```python
from build123d import *

# Parameters (mm, degrees)
SKETCH1_W            = 1447.8
SKETCH1_H            = 215.9
BOSS_EXTRUDE1_DEPTH  = 6.35
SKETCH2_R            = 82.55
CUT_EXTRUDE1_DEPTH   = 7.35
LPATTERN1_COUNT      = 7
LPATTERN1_PITCH      = 203.2
FILLET1_R            = 25.4
CUT_EXTRUDE2_DEPTH   = 7.35
LPATTERN2_COUNT      = 2
LPATTERN2_PITCH      = 406.4
MIRROR1_COPY_1_DEPTH = 7.35
SKETCH4_R            = 3.175
CUT_EXTRUDE3_DEPTH   = 7.35


with BuildPart() as part:
    # Sketch1 → Boss-Extrude1 (new body)
    with BuildSketch(Plane.XY):
        Rectangle(SKETCH1_W, SKETCH1_H)
    extrude(amount=BOSS_EXTRUDE1_DEPTH)

    # Sketch2 → Cut-Extrude1 (cut, through all)
    with BuildSketch(Plane.XY.offset(6.35)):
        with Locations((-609.6, 0)):
            Circle(SKETCH2_R)
    cut_extrude1 = extrude(amount=-CUT_EXTRUDE1_DEPTH, mode=Mode.SUBTRACT)

    # LPattern1: Cut-Extrude1 ×7
    with Locations(*[(i * LPATTERN1_PITCH, 0, 0) for i in range(1, LPATTERN1_COUNT)]):
        add(cut_extrude1, mode=Mode.SUBTRACT)

    # Fillet1
    fillet1_edges = [part.edges().sort_by_distance(p)[0] for p in [
        (-723.9, 107.95, 3.175),
        (723.9, 107.95, 3.175),
    ]]
    fillet(fillet1_edges, radius=FILLET1_R)

    # Sketch3 → Cut-Extrude2 (cut, through all)
    with BuildSketch(Plane.XY.offset(6.35)):
        with BuildLine():
            Line((-706.4375, 50.8), (-706.4375, 31.75))
            ThreePointArc((-706.4375, 31.75), (-711.2, 26.9875), (-715.9625, 31.75))
            Line((-715.9625, 31.75), (-715.9625, 50.8))
            ThreePointArc((-715.9625, 50.8), (-711.2, 55.5625), (-706.4375, 50.8))
        make_face()
    cut_extrude2 = extrude(amount=-CUT_EXTRUDE2_DEPTH, mode=Mode.SUBTRACT)

    # LPattern2: Cut-Extrude2 ×2
    with Locations(*[(i * LPATTERN2_PITCH, 0, 0) for i in range(1, LPATTERN2_COUNT)]):
        add(cut_extrude2, mode=Mode.SUBTRACT)

    # Mirror1: Cut-Extrude2 across plane
    add(cut_extrude2.mirror(Plane(origin=(0, 0, 0), x_dir=(0, 0, 1), z_dir=(1, 0, 0))), mode=Mode.SUBTRACT)

    # Mirror1 copy 1 sketch → Mirror1 copy 1 (cut, through all)
    with BuildSketch(Plane(origin=(-406.4, 0, 6.35), x_dir=(-1, 0, 0), z_dir=(0, 0, 1))):
        with BuildLine():
            Line((-706.4375, -50.8), (-706.4375, -31.75))
            ThreePointArc((-706.4375, -31.75), (-711.2, -26.9875), (-715.9625, -31.75))
            Line((-715.9625, -31.75), (-715.9625, -50.8))
            ThreePointArc((-715.9625, -50.8), (-711.2, -55.5625), (-706.4375, -50.8))
        make_face()
    extrude(amount=-MIRROR1_COPY_1_DEPTH, mode=Mode.SUBTRACT)

    # Sketch4 → Cut-Extrude3 (cut, through all)
    with BuildSketch(Plane.XY.offset(6.35)):
        with Locations((-698.5, 19.05)):
            Circle(SKETCH4_R)
        with Locations((-317.5, 19.05)):
            Circle(SKETCH4_R)
        with Locations((-292.1, 19.05)):
            Circle(SKETCH4_R)
        with Locations((-698.5, -82.55)):
            Circle(SKETCH4_R)
        with Locations((-317.5, -82.55)):
            Circle(SKETCH4_R)
        with Locations((-292.1, -82.55)):
            Circle(SKETCH4_R)
    cut_extrude3 = extrude(amount=-CUT_EXTRUDE3_DEPTH, mode=Mode.SUBTRACT)

    # Mirror2: Cut-Extrude3 across plane
    add(cut_extrude3.mirror(Plane(origin=(0, 0, 0), x_dir=(0, 0, 1), z_dir=(1, 0, 0))), mode=Mode.SUBTRACT)


solid = part.part
```
Read the model definition and answer for the solid it produces. Units are mm, in the model's axes. Coordinates: 2 decimals unless noted, no trailing zeros. Write each loop counter-clockwise with the first axis right and the second up, starting at its lowest first coordinate (ties: lowest second). Pieces come first, ordered by that corner, then holes. Notation, with made-up numbers: (19, 22.5) -> (76, 22.5) arc R11 ccw to (76, 38.5) -> close; hole circle Ø1 at (46.25, -27.5). An arc over 180 degrees is marked (long way). Answer as a JSON object with one key per item and string values.
Q1. The part is cut by section B-B on y = -43. Give the number of separate pieces and of enclosed holes in the cut face, then the cut area to 3 significant figures.
The answers:
{"separate pieces": "8", "enclosed holes": "0", "area": "2,930 mm2"}
Q2. The part is cut by section A-A on x = -406.4. Give the vertices of the cut face in (y, z).
The answers:
{"outline": "(-107.95, 0) -> (-82.55, 0) -> (-82.55, 6.35) -> (-107.95, 6.35) -> close; (82.55, 0) -> (107.95, 0) -> (107.95, 6.35) -> (82.55, 6.35) -> close"}
Q3. Determine the mould class of faces 1 (the flat face through (-10, -94, 6.35)), 2 (the cylindrical face through (716.26, 100.71, 3.22)), 3 (the cylindrical face through (482.655, -31.617, 3.219)), 4 (the cylindrical face through (-285.67, 3.63, 3.22)) for opening direction Y: pulls with the +Y half, pulls with the -Y half, needs draft (parallel to the pull), parting line crosses it, or undercut.
The answers:
{"face 1": "needs draft", "face 2": "pulls with the +Y half", "face 3": "undercut", "face 4": "undercut"}
Q4. Consider line 1 (Y direction, x = -292.1, z = 1.5) (3 decimals); line 2 (Y direction, x = 609.6, z = 3.25); line 3 (Y direction, x = -617, z = 4.25). Determine where each line is inside the solid, lowest interval first. Write a range as [from, to].
The answers:
{"line 1": "y = [-107.95, -85.725], [-79.375, 15.875], [22.225, 107.95]", "line 2": "y = [-107.95, -82.55], [82.55, 107.95]", "line 3": "y = [-107.95, -82.22], [82.22, 107.95]"}
Q5. The part is cut by section D-D on x = 136.5. Give the vertices of the cut face in (y, z), then the cut area to 3 significant figures.
The answers:
{"outline": "(-107.95, 0) -> (-48.64, 0) -> (-48.64, 6.35) -> (-107.95, 6.35) -> close; (48.64, 0) -> (107.95, 0) -> (107.95, 6.35) -> (48.64, 6.35) -> close", "area": "753 mm2"}
